Part model, mm, in its own coordinate system. A direction names the side the tool comes from. Coordinates: 2 decimals unless noted, no trailing zeros. Write each loop counter-clockwise with the first axis right and the second up, starting at its lowest first coordinate (ties: lowest second). Pieces come first, ordered by that corner, then holes. Notation, with made-up numbers: (61.5, -13) -> (73.5, -13) arc R19 cw to (73.5, 2) -> close; hole circle Ø2 at (-8, 67). An arc over 180 degrees is marked (long way). One line per question, with ' | ' between items. Start each with the question number.
Item 1: Saw through at C-C (x = 38.5). List the corners of the cut face in (y, z).
Item 2: Probe probe 1 along Z at (x, y) = (38.5, 88); probe 2 along Z at (x, y) = (25, 7.5); probe 3 along Y at (x, z) = (34.5, 4). List the from-to ranges inside material, lowest first. Write a range as [from, to].
Item 3: Two-plate mould, pull along Z, no slides. Class faces 1 (the flat face through (33, 0, 3)), 2 (the flat face through (33, 64, 0)), 3 (the flat face through (4, 63, 8.5)): pulls with the +Z half, pulls with the -Z half, needs draft (parallel to the pull), parting line crosses it, or undercut.
Item 4: Pin check, flat tips, straight feed: pin 1 (0.9 mm diameter, centred on y = 1, z = 4.5, fed in from -X); pin 2 (0.5 mm diameter, centred on x = 32.5, z = 4, fed in from -Y); pin 3 (0.6 mm diameter, centred on x = 32, y = 1, fed in from +Z). Stop position of each tip, or through.
Item 5: Saw through at A-A (y = 53). List the corners of the cut face in (x, z), and give its area (3 significant figures).
Item 6: 3-axis set-ups, long thin cutter, end or side, ignore diameter. For faces 4 (the flat face through (33, 63, 8.3)), 5 (the cylindrical face through (64.67, 123.8, 4.31)): which of +Z, -Z, +X, -X, +Y, -Y reach the whole face in a straight line?
Item 7: Saw through at B-B (x = 12). List the corners of the cut face in (y, z).
Autodesk Inventor part; units mm, degrees
ref_plane "YZ Plane" through (0, 0, 0) normal (1, 0, 0) x (0, 1, 0)
ref_plane "XZ Plane" through (0, 0, 0) normal (0, 1, 0) x (-1, 0, 0)
ref_plane "XY Plane" through (0, 0, 0) normal (0, 0, 1) x (1, 0, 0)
sketch "Skizze1" plane through (0, 0, 0) normal (0, 0, 1) x (1, 0, 0)
  line L0 (0, 0) -> (66.1, 0)
  line L1 (66.1, 0) -> (66.1, 125.3)
  line L2 (66.1, 125.3) -> (0, 125.3)
  line L3 (0, 125.3) -> (0, 0)
  dimension "d0" = 66.1
  dimension "d1" = 125.3
extrude "Extrusion1" add sketch "Skizze1" along normal blind 8.5
fillet "Rundung1" radius 5 1 edges at (66.1, 125.3, 4.25)
fillet "Rundung2" radius 5 1 edges at (0, 125.3, 4.25)
fillet "Rundung3" radius 5 1 edges at (0, 0, 4.25)
fillet "Rundung4" radius 5 1 edges at (66.1, 0, 4.25)
sketch "Skizze2" plane through (0, 0, 8.5) normal (0, 0, 1) x (1, 0, 0)
  line L0 (66.1, 5) -> (66.1, 120.3)
  line L1 (61.1, 125.3) -> (5, 125.3)
  line L2 (0, 120.3) -> (0, 5)
  line L3 (5.05, 109.15) -> (61.05, 109.15)
  line L4 (61.05, 109.15) -> (61.05, 16.15)
  line L5 (61.05, 16.15) -> (5.05, 16.15)
  line L6 (5.05, 16.15) -> (5.05, 109.15)
  point P0 (0, 0)
  dimension "d8" = 56
  dimension "d9" = 93
  dimension "d10" = 5.05
  dimension "d11" = 16.15
sketch "Skizze3" plane through (0, 0, 8.5) normal (0, 0, 1) x (1, 0, 0)
  line L0 (66.1, 5) -> (66.1, 120.3)
  line L1 (61.1, 125.3) -> (5, 125.3)
  line L2 (0, 120.3) -> (0, 5)
  line L3 (5, 0) -> (61.1, 0)
  circle A0 centre (12, 118.6) radius 1.5
  line L4 (25.9, 119.7) -> (40.2, 119.7)
  arc A1 (40.2, 118.3) -> (40.2, 119.7) centre (40.2, 119) ccw
  line L5 (40.2, 118.3) -> (25.9, 118.3)
  arc A2 (25.9, 119.7) -> (25.9, 118.3) centre (25.9, 119) ccw
  point P0 (0, 0)
  dimension "d0" = 66.1
  dimension "d12" = 6.7
  dimension "d13" = 12
  dimension "d14" = 3
  dimension "d19" = 1.4
  dimension "d22" = 5.6
  dimension "d23" = 15.7
  dimension "d27" = 14.3
  dimension "d28" = 25.9
extrude "Extrusion2" add sketch "Skizze3" along normal blind 0.2
extrude "Extrusion3" cut sketch "Skizze2" against normal blind 0.2
sketch "Skizze5" plane through (5, 0, 0) normal (0, -1, 0) x (1, 0, 0)
  line L0 (0, 8.5) -> (56.1, 8.5)
  line L1 (0, 0) -> (0, 8.5)
  line L2 (0, 0) -> (56.1, 0)
  line L3 (24.575, 5.15) -> (31.425, 5.15)
  line L4 (31.425, 5.15) -> (31.425, 3.35)
  line L5 (31.425, 3.35) -> (24.575, 3.35)
  line L6 (24.575, 3.35) -> (24.575, 5.15)
  line L7 (56.1, 8.5) -> (56.1, 0)
  line L8 (0, 8.5) -> (56.1, 8.5)
  line L9 (0, 0) -> (0, 8.5)
  line L10 (0, 0) -> (56.1, 0)
  point P0 (-5, 0)
  dimension "d33" = 6.85
  dimension "d34" = 1.8
  dimension "d35" = 24.575
  dimension "d36" = 3.35
extrude "Extrusion4" cut sketch "Skizze5" against normal blind 2 contours L3 L4 L5 L6
equation "\"d10\" = -0.5 * d8 + 0.5 * d0"
equation "\"d11\" = -0.5 * d9 + 0.5 * d1"
equation "\"d28\" = 0.5 * d0 - 0.5 * d27"
equation "\"d35\" = -0.5 * d33 + 0.5 * d8"
properties part number "Galaxy S2"
From the geometry:
1) outline: (0, 0) -> (125.3, 0) -> (125.3, 8.5) -> (119.7, 8.5) -> (119.7, 8.7) -> (118.3, 8.7) -> (118.3, 8.5) -> (109.15, 8.5) -> (109.15, 8.3) -> (16.15, 8.3) -> (16.15, 8.5) -> (0, 8.5) -> close
2) probe 1: [0, 8.3] | probe 2: [0, 8.5] | probe 3: [2, 125.3]
3) face 1: needs draft | face 2: pulls with the -Z half | face 3: pulls with the +Z half
4) pin 1: x = 1.48 | pin 2: y = 2 | pin 3: z = 8.5
5) outline: (0, 0) -> (66.1, 0) -> (66.1, 8.5) -> (61.05, 8.5) -> (61.05, 8.3) -> (5.05, 8.3) -> (5.05, 8.5) -> (0, 8.5) -> close | area: 551 mm2
6) face 4: +Z | face 5: +Z, -Z, +X, +Y
7) outline: (0, 0) -> (125.3, 0) -> (125.3, 8.5) -> (120.1, 8.5) -> (120.1, 8.7) -> (117.1, 8.7) -> (117.1, 8.5) -> (109.15, 8.5) -> (109.15, 8.3) -> (16.15, 8.3) -> (16.15, 8.5) -> (0, 8.5) -> close
